Geometry check sheet. Reference: the model listing, model coordinates, mm. Round coordinates to 2 decimals unless told otherwise and drop trailing zeros. Order: outer loops, then holes, each group sorted by start corner. A loop starts at its lowest first (then second) coordinate and runs counter-clockwise, first axis right, second up. Notation, with made-up numbers: (37.25, 43) - (83.25, 43) arc R24 cw to (83.25, 69) - close; hole circle Ø8 at (-11, 79). An arc over 180 degrees is marked (long way). Return JSON: item names as keys, results as strings. Group by question number.
Q1. Draft check along X on faces 1 (the flat face through (46, 1, 0)), 2 (the cylindrical face through (11.923, -3.755, 1.479)). Enter one of: pulls with the +X half, pulls with the -X half, needs draft (parallel to the pull), parting line crosses it, or undercut.
Q2. Material ranges on line 1 along Y through (x, z) = (0, 1.2); line 2 along X through (y, z) = (10, 2.05); line 3 along Y through (x, z) = (-43.5, 1.95), recorded low to high.
Q3. Sectioned sample at A-A, the plane x = 0. Record the cut outline in (y, z), then the cut area to 3 significant figures.
Q4. Sectioned sample at D-D, the plane x = 135.5. Record the cut outline in (y, z), then the cut area to 3 significant figures.
Q5. Sectioned sample at C-C, the plane z = 2.5. Record the cut outline in (x, y), then the cut area to 3 significant figures.
Q6. Gauge pin test, flat ends, axial feed: pin 1 Ø0.7 at (y, z) = (-33.5, 1.5) entering from -X; pin 2 Ø0.7 at (y, z) = (33, 1.5) entering from -X; pin 3 Ø1.5 at (x, z) = (-48.5, 1) entering from -Y. Record the tip position at first contact, or that the pin passes through.
Q7. Sectioned sample at B-B, the plane y = 0. Record the cut outline in (x, z).
```python
from build123d import *

# Parameters (mm, degrees)
F1_DEPTH = 3


with BuildPart() as f1:
    # F0 (on Top) → F1 (new body)
    with BuildSketch(Plane.XY):
        with BuildLine():
            ThreePointArc((30.199338, 32), (0, 44), (-30.199338, 32))
            Line((-30.199338, 32), (-54.820662, 32))
            Line((-54.820662, 32), (-54.820662, 0))
            Line((-54.820662, 0), (-54.820662, -32))
            Line((-54.820662, -32), (-30.199338, -32))
            ThreePointArc((-30.199338, -32), (0, -44), (30.199338, -32))
            Line((30.199338, -32), (57.179338, -32))
            Line((57.179338, -32), (57.179338, -34.461271))
            Line((57.179338, -34.461271), (150.179338, -34.461271))
            Line((150.179338, -34.461271), (150.179338, 0))
            Line((150.179338, 0), (150.179338, 34.461271))
            Line((150.179338, 34.461271), (57.179338, 34.461271))
            Line((57.179338, 34.461271), (57.179338, 32))
            Line((57.179338, 32), (30.199338, 32))
        make_face()
        with BuildLine():
            ThreePointArc((-12.5, 0), (0, 12.5), (12.5, 0))
            ThreePointArc((12.5, 0), (0, -12.5), (-12.5, 0))
        make_face(mode=Mode.SUBTRACT)
    extrude(amount=F1_DEPTH)


solid = f1.part
```
Reply:
{
 "1": {"face 1": "needs draft", "face 2": "undercut"},
 "2": {"line 1": "-44 to -12.5, 12.5 to 44", "line 2": "-54.82 to -7.5, 7.5 to 150.18", "line 3": "-32 to 32"},
 "3": {"outline": "(-44, 0) - (-12.5, 0) - (-12.5, 3) - (-44, 3) - close; (12.5, 0) - (44, 0) - (44, 3) - (12.5, 3) - close", "area": "189 mm^2"},
 "4": {"outline": "(-34.46, 0) - (34.46, 0) - (34.46, 3) - (-34.46, 3) - close", "area": "207 mm^2"},
 "5": {"outline": "(-54.82, -32) - (-30.2, -32) arc R44 ccw to (30.2, -32) - (57.18, -32) - (57.18, -34.46) - (150.18, -34.46) - (150.18, 34.46) - (57.18, 34.46) - (57.18, 32) - (30.2, 32) arc R44 ccw to (-30.2, 32) - (-54.82, 32) - close; hole circle Ø25 at (0, 0)", "area": "14,100 mm^2"},
 "6": {"pin 1": "x = -28.93", "pin 2": "x = -29.5", "pin 3": "y = -32"},
 "7": {"outline": "(-54.82, 0) - (-12.5, 0) - (-12.5, 3) - (-54.82, 3) - close; (12.5, 0) - (150.18, 0) - (150.18, 3) - (12.5, 3) - close"}
}
